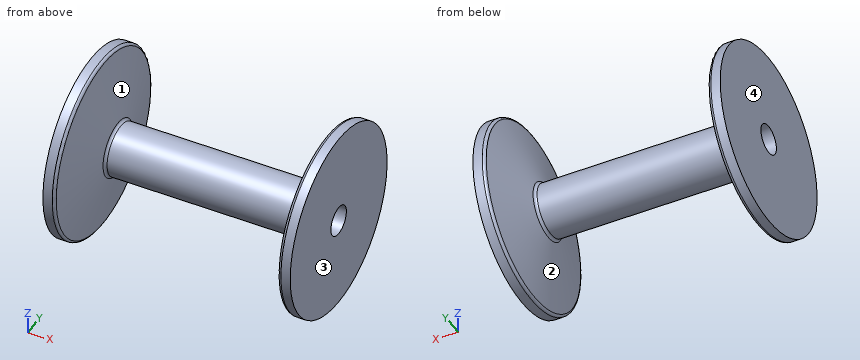
from build123d import *


with BuildPart() as f1:
    # F0 (on Front) → F1 (revolve)
    with BuildSketch(Plane.XZ):
        with BuildLine():
            Line((0, 5.1), (42.5, 5.1))
            Line((42.5, 5.1), (42.5, 31.95))
            Line((42.5, 31.95), (39.295436, 31.95))
            ThreePointArc((39.295436, 31.95), (38.672921, 31.732608), (38.321066, 31.174951))
            Line((38.321066, 31.174951), (33.380509, 9.775049))
            ThreePointArc((33.380509, 9.775049), (33.028654, 9.217392), (32.406139, 9))
            Line((32.406139, 9), (0, 9))
            Line((0, 9), (-32.406139, 9))
            ThreePointArc((-32.406139, 9), (-33.028654, 9.217392), (-33.380509, 9.775049))
            Line((-33.380509, 9.775049), (-38.321066, 31.174951))
            ThreePointArc((-38.321066, 31.174951), (-38.672921, 31.732608), (-39.295436, 31.95))
            Line((-39.295436, 31.95), (-42.5, 31.95))
            Line((-42.5, 31.95), (-42.5, 5.1))
            Line((-42.5, 5.1), (0, 5.1))
        make_face()
    revolve(axis=Axis((21.25, 0, 0), (1, 0, 0)))


solid = f1.part
Model file for the job. Use its own axes, mm. Face numbers are marked on the shaded views. Give positions to 0.01 mm unless a question says otherwise; leave off trailing zeros. Order: outer loops, then holes, each group sorted by start corner. A loop starts at its lowest first (then second) coordinate and runs counter-clockwise, first axis right, second up. Notation, with made-up numbers: M 71.5,-27.5 L 75.5,-27.5 A35 ccw 75.5,5.5 Z; hole C 80.5,30.5 d11. An arc over 180 degrees is marked long. Put each result on its own line as item: value. Start each with the question number.
(1) Band-saw the part on A-A on y = 0. Give the cut face in (x, z), then the cut area to 3 significant figures.
(2) Drill centre lines: L1, parallel to Y at x = 1, z = 0; L2, parallel to X at y = -13.5, z = -28. Where is each one in solid material? Low to high. Write a range as [from, to].
(3) Pin check, flat tips, straight feed: pin 1 Ø10 at (x, y) = (12, 0.5) entering from -Z; pin 2 Ø5 at (x, y) = (19.5, -8.5) entering from +Z; pin 3 Ø8 at (x, z) = (10.5, 14.5) entering from -Y; pin 4 Ø3 at (x, z) = (-14, -4) entering from -Y. Stop position of each tip, or through.
(4) Band-saw the part on C-C on x = 1. Give the cut face in (y, z).
(5) Pull direction X, two halves, no side cores. Call the marked faces 1, 2, 3 and 4: released by +X, released by -X, zero draft, split by the parting line, or undercut.
Results below:
1. outline: M -42.5,-31.95 L -39.3,-31.95 A1 ccw -38.32,-31.17 L -33.38,-9.78 A1 cw -32.41,-9 L 32.41,-9 A1 cw 33.38,-9.78 L 38.32,-31.17 A1 ccw 39.3,-31.95 L 42.5,-31.95 L 42.5,-5.1 L -42.5,-5.1 Z; M -42.5,5.1 L 42.5,5.1 L 42.5,31.95 L 39.3,31.95 A1 ccw 38.32,31.17 L 33.38,9.78 A1 cw 32.41,9 L -32.41,9 A1 cw -33.38,9.78 L -38.32,31.17 A1 ccw -39.3,31.95 L -42.5,31.95 Z
1. area: 1,270 mm2
2. L1: y = [-9, -5.1], [5.1, 9]
2. L2: x = [-42.5, -38.3], [38.3, 42.5]
3. pin 1: stops at z = -9
3. pin 2: stops at z = 6.71
3. pin 3: passes through
3. pin 4: stops at y = -8.65
4. outline: C 0,0 d18; hole C 0,0 d10.2
5. face 1: undercut
5. face 2: undercut
5. face 3: released by +X
5. face 4: released by -X
